Here's how the part is built. I have some questions about the finished solid (model axes, mm). A direction names the side the tool comes from. Coordinates: 2 decimals unless noted, no trailing zeros. Loops run counter-clockwise (first coordinate to the right, second up) from the corner with the lowest first, then second, coordinate; pieces in that order, holes last. Notation, with made-up numbers: (32, -36) - (89, -36) arc R23 ccw to (89, -13) - close; hole circle Ø4 at (60.25, 6.25). An arc over 180 degrees is marked (long way). Use a Markdown table: item, result.
```python
from build123d import *

# Parameters (mm, degrees)
EXTRUDE_1_DEPTH     = 40
SKETCH_2_R          = 5
CUT_EXTRUDE_1_DEPTH = 148.24755879


with BuildPart() as part:
    # 草图1 → 凸台-拉伸1 (new body)
    with BuildSketch(Plane.XY):
        Polygon((0, 0), (-137.873085422, 24.310744873), (-136.136603645, 34.158822403), (0, 10.154266119), (136.136603645, 34.158822403), (137.873085422, 24.310744873), align=None)
    extrude(amount=EXTRUDE_1_DEPTH)

    # 草图2 → 切除-拉伸1 (cut, through all)
    with BuildSketch(Plane(origin=(1.736481777, 9.84807753, 0), x_dir=(0.984807753012208, -0.17364817766693144, 0), z_dir=(0.17364817766693144, 0.984807753012208, 0))):
        with Locations(Location((-41.763269807, -20, 0), (0, 0, 180))):
            Circle(SKETCH_2_R)
        with Locations(Location((-101.763269807, -20, 0), (0, 0, 180))):
            Circle(SKETCH_2_R)
    cut_extrude_1 = extrude(amount=-CUT_EXTRUDE_1_DEPTH, mode=Mode.SUBTRACT)

    # 镜向1: 切除-拉伸1 across plane
    add(cut_extrude_1.mirror(Plane(origin=(0, 0, 0), x_dir=(0, 0, 1), z_dir=(1, 0, 0))), mode=Mode.SUBTRACT)


solid = part.part
```
Q1. Please list where these lines run through material, in increasing order: L1, parallel to Y at x = -37, z = 32.5; L2, parallel to Y at x = 13, z = 10. Write a range as from..to.
Check values:
| item | result |
|---|---|
| L1 | 6.52..16.68 |
| L2 | 2.29..12.45 |
Q2. I want a section at D-D, the plane y = 4. Write out the boundary of the cut face in (x, z), then the cut area to 3 significant figures.
Check values:
| item | result |
|---|---|
| outline | (-22.69, 0) - (22.69, 0) - (22.69, 40) - (-22.69, 40) - close |
| area | 1,810 mm^2 |
Q3. Will these pins go through, and if not, where does the flat tip stop? P1, Ø1, axis at x = 92, z = 8.5, coming from the +Y side; P2, Ø5, axis at x = 65, z = 30.5, coming from the +Y side; P3, Ø1.5, axis at x = 43, y = 19.5, coming from the +Z side; P4, Ø5, axis at x = -34.5, z = 26, coming from the +Y side.
Check values:
| item | result |
|---|---|
| P1 | y = 26.46 |
| P2 | y = 22.06 |
| P3 | through |
| P4 | y = 16.68 |
Q4. I want a section at A-A, the plane y = 22. Give the number of separate pieces and of enclosed holes in the cut face, then the cut area to 3 significant figures.
Check values:
| item | result |
|---|---|
| separate pieces | 2 |
| enclosed holes | 2 |
| area | 4,450 mm^2 |
Q5. I want a section at C-C, the plane x = 64.5. Write out the boundary of the cut face in (y, z), then the cut area to 3 significant figures.
Check values:
| item | result |
|---|---|
| outline | (11.37, 0) - (21.53, 0) - (21.53, 40) - (11.37, 40) - close |
| area | 406 mm^2 |
Q6. I want a section at B-B, the plane z = 8. Write out the boundary of the cut face in (x, y).
Check values:
| item | result |
|---|---|
| outline | (-137.87, 24.31) - (0, 0) - (137.87, 24.31) - (136.14, 34.16) - (0, 10.15) - (-136.14, 34.16) - close |
Q7. If we mould it in two halves opening along X, with no side actions, what happens to faces 3 (the face through (-69.021, 22.325, 19.72)), 4 (the face through (-137.017, 29.166, 19.72)), 5 (the face through (136.993, 29.304, 19.72)), 6 (the face through (-101.609, 23.065, 15.564))? For each: pulls with the +X half, pulls with the -X half, needs draft (parallel to the pull), parting line crosses it, or undercut.
Check values:
| item | result |
|---|---|
| face 3 | undercut |
| face 4 | pulls with the -X half |
| face 5 | pulls with the +X half |
| face 6 | undercut |
Q8. Which directions (+Z, -Z, +X, -X, +Y, -Y) give clear straight access to the entire face, cutting with the end or side of a thin tool? Please do faces 1 (the face through (69.902, 12.326, 19.72)), 2 (the face through (67.12, 21.99, 19.72)).
Check values:
| item | result |
|---|---|
| face 1 | +Z, -Z, +X, -Y |
| face 2 | +Z, -Z, +Y |
